Could you check a few things on this model? Use its own coordinates, in mm. Face numbers are marked on the shaded views. A direction names the side the tool comes from. Round coordinates to 2 decimals unless told otherwise and drop trailing zeros. Loops run counter-clockwise (first coordinate to the right, second up) from the corner with the lowest first, then second, coordinate; pieces in that order, holes last. Notation, with made-up numbers: (-32.5, -2.75) -> (-4.5, -2.75) arc R19 cw to (-4.5, 10.25) -> close; hole circle Ø11 at (-32.75, 69). An arc over 180 degrees is marked (long way). Put each result on its own line as item: value. Start each with the question number.
1. I'm going to push flat-ended pins straight in: P1, Ø6.5, axis at y = 4.5, z = 1, coming from the -X side; P2, Ø1, axis at y = 13.5, z = 8.5, coming from the -X side; P3, Ø2, axis at x = -15, y = 20, coming from the -Z side; P4, Ø10, axis at y = 7.5, z = -5, coming from the +X side. Where does each tip first touch, or does it pass through?
2. Imagine slicing it at B-B, the plane y = 23. Please give me the cut outline in (x, z).
3. Which directions (+Z, -Z, +X, -X, +Y, -Y) give clear straight access to the entire face, cutting with the end or side of a thin tool? Please do the marked faces 1 and 2.
4. I need wall thicknesses on line 1 (Z direction, x = -0.5, y = 8); line 2 (X direction, y = 18, z = 7.5); line 3 (Z direction, x = -17, y = -1.5). Which ranges of each line are inside material? Lowest first, please. Write a range as [from, to].
5. If we mould it in two halves opening along Y, with no side actions, what happens to the marked faces 3, 4 and 5? For each: pulls with the +Y half, pulls with the -Y half, needs draft (parallel to the pull), parting line crosses it, or undercut.
6. Imagine slicing it at A-A, the plane x = -28. Please give me the cut outline in (y, z).
```python
from build123d import *

# Parameters (mm, degrees)
SKETCH3_R   = 13.7795
SKETCH3_R_2 = 7.8994


with BuildPart() as part:
    # Sketch1 → Revolve1 (revolve)
    with BuildSketch(Plane.XY, mode=Mode.PRIVATE) as revolve1_sk:
        Polygon((-31.75, -13.7795), (-12.7, -13.7795), (-12.7, -10.6172), (-31.75, -10.7696), align=None)
    revolve(revolve1_sk.sketch.rotate(Axis((-31.75, 0, 0), (1, 0, 0)), 270), axis=Axis((-31.75, 0, 0), (1, 0, 0)))


with BuildPart() as body_2:
    # Sketch2 → Revolve2 (revolve)
    with BuildSketch(Plane.XY, mode=Mode.PRIVATE) as revolve2_sk:
        Polygon((10.7696, 31.75), (10.6172, 12.7), (13.7795, 12.7), (13.7795, 31.75), align=None)
    revolve(revolve2_sk.sketch.rotate(Axis((0, 0, 0), (0, 1, 0)), 90), axis=Axis((0, 0, 0), (0, 1, 0)))


with BuildPart() as sweep1_tool:
    # Sweep1: sweep along a path in Sketch4
    with BuildLine(Plane.XY) as sweep1_path:
        ThreePointArc((-12.7, 0), (-3.719744, 3.719744), (0, 12.7))
    # Sketch3 → Sweep1 (sweep)
    with BuildSketch(Plane(origin=(-12.7, 0, 0), x_dir=(0, 0, -1), z_dir=(1, 0, 0))):
        Circle(SKETCH3_R)
        Circle(SKETCH3_R_2, mode=Mode.SUBTRACT)
    sweep(path=sweep1_path.line)


with BuildPart() as part_1:
    add(part.part)


with BuildPart() as part_2:
    # Sweep1: joined with sweep1_tool
    add(part_1.part.fuse(sweep1_tool.part, body_2.part, tol=0.00001))


solid = part_2.part
```
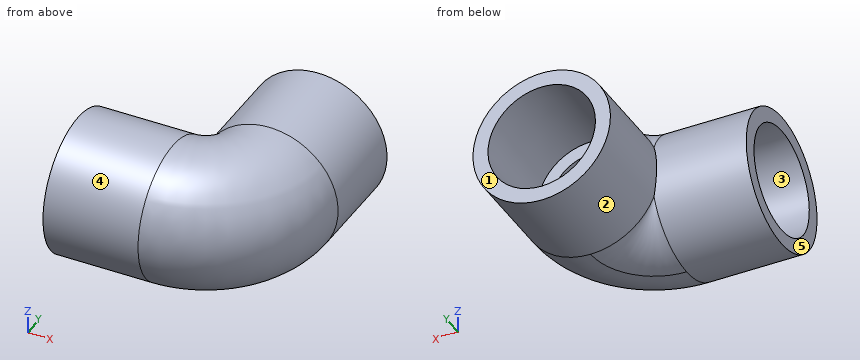
Entries:
1. P1: x = 4.17
1. P2: x = -11.22
1. P3: through
1. P4: x = 13.66
2. outline: circle Ø27.56 at (0, 0); hole circle Ø21.4 at (0, 0)
3. face 1: +Z, -Z, +X, -X, +Y
3. face 2: +Y
4. line 1: [-13.77, -7.89], [7.89, 13.77]
4. line 2: [-11.56, -7.57], [7.57, 11.56]
4. line 3: [-13.7, -10.55], [10.55, 13.7]
5. face 3: undercut
5. face 4: parting line crosses it
5. face 5: needs draft
6. outline: circle Ø27.56 at (0, 0); hole circle Ø21.48 at (0, 0)
